Could you check a few things on this model? Use its own coordinates, in mm. Give positions to 0.01 mm unless a question says otherwise; leave off trailing zeros. Loops run counter-clockwise (first coordinate to the right, second up) from the corner with the lowest first, then second, coordinate; pieces in that order, holes last. Notation, with made-up numbers: (-32.75, 26) -> (-27.75, 26) arc R16 ccw to (-27.75, 49) -> close; hole circle Ø6 at (67.25, 87). An arc over 180 degrees is marked (long way). Write each question's results on one line, items separated by ' | '. Start each with the question number.
Q1. If I drill on line 1 along X through (y, z) = (3.25, 16); line 2 along Y through (x, z) = (5.6, 10.5); line 3 along X through (y, z) = (7.5, 47), over which ranges is the centre line in solid material (lowest first)?
Q2. If we section it at C-C, the plane y = 3: List the corners of the cut face in (x, z) for me, plus the area to 3 significant figures.
Q3. If we section it at B-B, the plane z = 60.5: List the corners of the cut face in (x, y) for me, plus the area to 3 significant figures.
Q4. Will these pins go through, and if not, where does the flat tip stop? P1, Ø3, axis at x = -5.6, y = 3, coming from the +Z side; P2, Ø4, axis at x = 2.5, z = 22, coming from the -Y side; P3, Ø1.2, axis at x = 6, y = 2, coming from the -Z side.
Q5. If we section it at A-A, the plane x = -5.6: List the corners of the cut face in (y, z) for me, plus the area to 3 significant figures.
Solid Edge part; units mm, degrees
sketch "Sketch1" plane through (0, 0, 0) normal (0, 0, 1) x (1, 0, 0)
  line L0 (8.6, 0) -> (8.6, 12.8)
  line L1 (8.6, 12.8) -> (3.6, 12.8)
  line L2 (3.6, 12.8) -> (3.6, 6)
  line L3 (3.6, 6) -> (-3.6, 6)
  line L4 (-3.6, 6) -> (-3.6, 12.8)
  line L5 (-3.6, 12.8) -> (-8.6, 12.8)
  line L6 (-8.6, 12.8) -> (-8.6, 0)
  line L7 (-8.6, 0) -> (8.6, 0)
extrude "Protrusion1" add sketch "Sketch1" along normal blind 200
sketch "Sketch2" plane through (0, 5.9, 200) normal (0, 0, 1) x (1, 0, 0)
  circle A0 centre (-5.6, -2.9) radius 2
  circle A1 centre (5.6, -2.9) radius 2
extrude "ExtrudedCutout_1" cut sketch "Sketch2" against normal blind 20
sketch "Sketch3" plane through (0, 5.9, 0) normal (0, 0, -1) x (-1, 0, 0)
  circle A0 centre (-5.6, -2.9) radius 2
  circle A1 centre (5.6, -2.9) radius 2
extrude "ExtrudedCutout_2" cut sketch "Sketch3" against normal blind 20
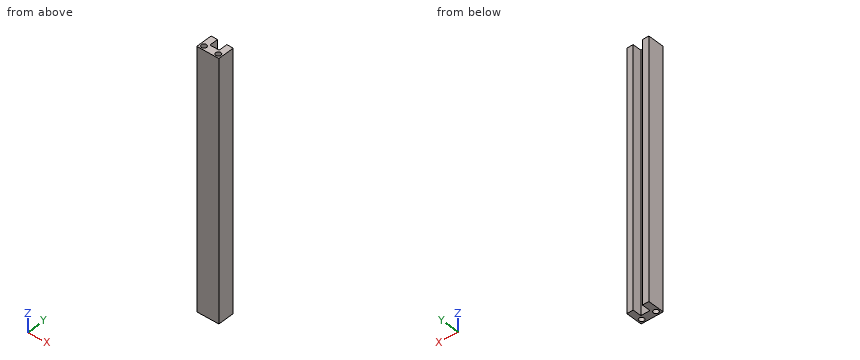
Final values:
1) line 1: x = -8.6 to -7.58, -3.62 to 3.62, 7.58 to 8.6 | line 2: y = 0 to 1, 5 to 12.8 | line 3: x = -8.6 to -3.6, 3.6 to 8.6
2) outline: (-8.6, 0) -> (-7.6, 0) -> (-7.6, 20) -> (-3.6, 20) -> (-3.6, 0) -> (3.6, 0) -> (3.6, 20) -> (7.6, 20) -> (7.6, 0) -> (8.6, 0) -> (8.6, 200) -> (7.6, 200) -> (7.6, 180) -> (3.6, 180) -> (3.6, 200) -> (-3.6, 200) -> (-3.6, 180) -> (-7.6, 180) -> (-7.6, 200) -> (-8.6, 200) -> close | area: 3,120 mm²
3) outline: (-8.6, 0) -> (8.6, 0) -> (8.6, 12.8) -> (3.6, 12.8) -> (3.6, 6) -> (-3.6, 6) -> (-3.6, 12.8) -> (-8.6, 12.8) -> close | area: 171 mm²
4) P1: stops at z = 180 | P2: stops at y = 0 | P3: stops at z = 20
5) outline: (0, 0) -> (1, 0) -> (1, 20) -> (5, 20) -> (5, 0) -> (12.8, 0) -> (12.8, 200) -> (5, 200) -> (5, 180) -> (1, 180) -> (1, 200) -> (0, 200) -> close | area: 2,400 mm²
